Can you work these out from the model? Positions are in its coordinate system, mm. Face numbers are marked on the shaded views. A direction names the side the tool comes from. Round coordinates to 2 decimals unless told otherwise and drop trailing zeros. Write each loop counter-clockwise with the first axis right and the second up, starting at its lowest first coordinate (ties: lowest second). Pieces come first, ordered by that corner, then holes. Notation, with made-up numbers: M 75,-21 L 118,-21 A15 ccw 118,-6 Z; hole C 52.25,-2.75 d10. An arc over 180 degrees is marked long. Answer as a JSON object with one key per item and string values. Group by question number.
1) Suppose I cut it at A-A, the plane x = 0. Write out the boundary of the cut face in (y, z), and give its area (3 significant figures).
2) On a 3-axis mill with a long thin cutter (end or side, diameter ignored), from which of +Z, -Z, +X, -X, +Y, -Y can I reach the whole of each face in a straight line? I mean the marked faces 5, 6 and 7. Say none if no direction works.
3) Suppose I cut it at B-B, the plane y = -30.5. Write out the boundary of the cut face in (x, z), and give its area (3 significant figures).
4) If we mould it in two halves opening along X, with no side actions, what happens to the marked faces 1, 2, 3 and 4? For each: +X half, -X half, draft (parallel to the pull), parting line (faces both ways), or undercut.
5) Suppose I cut it at C-C, the plane x = 52.5. Write out the boundary of the cut face in (y, z), and give its area (3 significant figures).
6) Suppose I cut it at D-D, the plane z = 17.5. State how many separate pieces and enclosed holes the cut face has, and give its area (3 significant figures).
7) I'm going to push flat-ended pins straight in: pin 1 Ø2 at (y, z) = (-42, 16.5) entering from -X; pin 2 Ø5 at (x, z) = (66.5, 18) entering from +Y; pin 3 Ø4.5 at (y, z) = (-80.16, 12.5) entering from -X. Where does each tip first touch, or does it pass through?
8) Please list where these lines run through material, in increasing order: L1, parallel to X at y = -78, z = 15.5; L2, parallel to X at y = -1, z = 32; L3, parallel to Y at x = -38, z = 25.5. Write a range as [from, to].
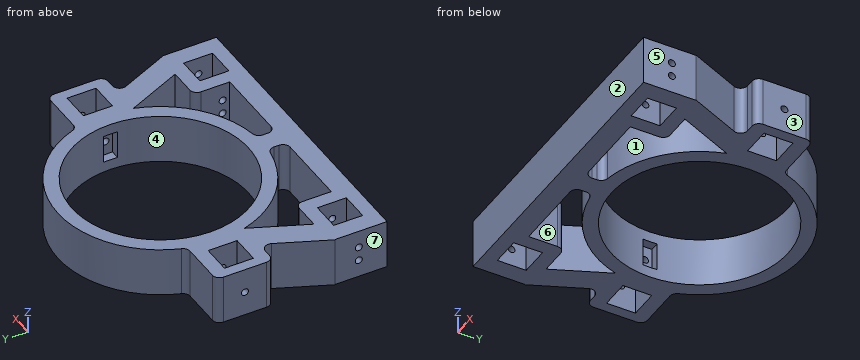
from build123d import *

# Parameters (mm, degrees)
SKETCH1_W                = 20.5
SKETCH1_H                = 20.5
SKETCH1_R                = 62.5
BOSS_EXTRUDE1_DEPTH      = 35
FILLET2_R                = 5
SKETCH2_W                = 20
SKETCH2_H                = 10
CUT_EXTRUDE2_DEPTH       = 7
SKETCH3_W                = 20
SKETCH3_H                = 10
CUT_EXTRUDE3_DEPTH       = 7
SKETCH4_W                = 35
SKETCH4_H                = 37
CUT_EXTRUDE4_DEPTH       = 10
SKETCH5_W                = 35
SKETCH5_H                = 37
CUT_EXTRUDE5_DEPTH       = 10
SKETCH6_W                = 35
SKETCH6_H                = 40.5
CUT_EXTRUDE8_DEPTH       = 2.5
SKETCH7_W                = 35
SKETCH7_H                = 40.5
CUT_EXTRUDE9_DEPTH       = 2.5
FILLET3_R                = 5
SKETCH8_R                = 2.5
CUT_EXTRUDE10_DEPTH      = 194
CUT_EXTRUDE10_DEPTH_BACK = 48
SKETCH9_R                = 2.5
CUT_EXTRUDE11_DEPTH      = 48
CUT_EXTRUDE11_DEPTH_BACK = 48
SKETCH10_R               = 2.5
CUT_EXTRUDE12_DEPTH      = 48
CUT_EXTRUDE12_DEPTH_BACK = 48


with BuildPart() as part:
    # Sketch1 → Boss-Extrude1 (new body)
    with BuildSketch(Plane.XY):
        with BuildLine():
            Line((117, -100.161277705), (117, -85.161277705))
            Line((117, -85.161277705), (88.226517383, -20.181680312))
            Line((88.226517383, -20.181680312), (108.734784021, -20.181680312))
            Line((108.734784021, -20.181680312), (108.734784021, 20.318319688))
            Line((108.734784021, 20.318319688), (69.594654141, 20.318319688))
            ThreePointArc((69.594654141, 20.318319688), (0, 72.5), (-69.594654141, 20.318319688))
            Line((-69.594654141, 20.318319688), (-108.734784021, 20.318319688))
            Line((-108.734784021, 20.318319688), (-108.734784021, -20.181680312))
            Line((-108.734784021, -20.181680312), (-88.226517383, -20.181680312))
            Line((-88.226517383, -20.181680312), (-117, -85.161277705))
            Line((-117, -85.161277705), (-117, -100.161277705))
            Line((-117, -100.161277705), (117, -100.161277705))
        make_face()
        with Locations((83.958397156, -79.911277705)):
            Rectangle(SKETCH1_W, SKETCH1_H, mode=Mode.SUBTRACT)
        with Locations((-83.958397156, -79.911277705)):
            Rectangle(SKETCH1_W, SKETCH1_H, mode=Mode.SUBTRACT)
        with BuildLine():
            Line((-63.708397156, -59.661277705), (-87.116280609, -59.661277705))
            Line((-87.116280609, -59.661277705), (-69.634400836, -20.181680312))
            ThreePointArc((-69.634400836, -20.181680312), (-46.29986484, -55.79043391), (-7, -72.161277705))
            Line((-7, -72.161277705), (-7, -85.161277705))
            Line((-7, -85.161277705), (-63.708397156, -85.161277705))
            Line((-63.708397156, -85.161277705), (-63.708397156, -59.661277705))
        make_face(mode=Mode.SUBTRACT)
        with BuildLine():
            Line((87.116280609, -59.661277705), (63.708397156, -59.661277705))
            Line((63.708397156, -59.661277705), (63.708397156, -85.161277705))
            Line((63.708397156, -85.161277705), (7, -85.161277705))
            Line((7, -85.161277705), (7, -72.161277705))
            ThreePointArc((7, -72.161277705), (46.29986484, -55.79043391), (69.634400836, -20.181680312))
            Line((69.634400836, -20.181680312), (87.116280609, -59.661277705))
        make_face(mode=Mode.SUBTRACT)
        with Locations((-88.484784021, 0.068319688)):
            Rectangle(SKETCH1_W, SKETCH1_H, mode=Mode.SUBTRACT)
        Circle(SKETCH1_R, mode=Mode.SUBTRACT)
        with Locations((88.484784021, 0.068319688)):
            Rectangle(SKETCH1_W, SKETCH1_H, mode=Mode.SUBTRACT)
    extrude(amount=BOSS_EXTRUDE1_DEPTH)

    # Fillet2
    fillet2_edges = [part.edges().sort_by_distance(p)[0] for p in [
        (-88.226517383, -20.181680312, 17.5),
        (-69.594654141, 20.318319688, 17.5),
        (69.594654141, 20.318319688, 17.5),
        (88.226517383, -20.181680312, 17.5),
        (7, -72.161277705, 17.5),
        (7, -85.161277705, 17.5),
        (63.708397156, -59.661277705, 17.5),
        (-63.708397156, -59.661277705, 17.5),
        (-7, -85.161277705, 17.5),
        (-7, -72.161277705, 17.5),
    ]]
    fillet(fillet2_edges, radius=FILLET2_R)

    # Sketch2 → Cut-Extrude2 (cut)
    with BuildSketch(Plane(origin=(61.7, 0, 0), x_dir=(0, 0, -1), z_dir=(1, 0, 0))):
        with Locations((-17.5, 0.068319688)):
            Rectangle(SKETCH2_W, SKETCH2_H)
    extrude(amount=CUT_EXTRUDE2_DEPTH, mode=Mode.SUBTRACT)

    # Sketch3 → Cut-Extrude3 (cut)
    with BuildSketch(Plane(origin=(-61.7, 0, 0), x_dir=(0, 0, -1), z_dir=(1, 0, 0))):
        with Locations((-17.5, 0.068319688)):
            Rectangle(SKETCH3_W, SKETCH3_H)
    extrude(amount=-CUT_EXTRUDE3_DEPTH, mode=Mode.SUBTRACT)

    # Sketch4 → Cut-Extrude4 (cut)
    with BuildSketch(Plane(origin=(117, 0, 0), x_dir=(0, 0, -1), z_dir=(1, 0, 0))):
        with Locations((-17.5, -81.661277705)):
            Rectangle(SKETCH4_W, SKETCH4_H)
    extrude(amount=-CUT_EXTRUDE4_DEPTH, mode=Mode.SUBTRACT)

    # Sketch5 → Cut-Extrude5 (cut)
    with BuildSketch(Plane.ZY.offset(117)):
        with Locations((17.5, -81.661277705)):
            Rectangle(SKETCH5_W, SKETCH5_H)
    extrude(amount=-CUT_EXTRUDE5_DEPTH, mode=Mode.SUBTRACT)

    # Sketch6 → Cut-Extrude8 (cut)
    with BuildSketch(Plane(origin=(108.734784021, 0, 0), x_dir=(0, 0, -1), z_dir=(1, 0, 0))):
        with Locations((-17.5, 0.068319688)):
            Rectangle(SKETCH6_W, SKETCH6_H)
    extrude(amount=-CUT_EXTRUDE8_DEPTH, mode=Mode.SUBTRACT)

    # Sketch7 → Cut-Extrude9 (cut)
    with BuildSketch(Plane.ZY.offset(108.734784021)):
        with Locations((17.5, 0.068319688)):
            Rectangle(SKETCH7_W, SKETCH7_H)
    extrude(amount=-CUT_EXTRUDE9_DEPTH, mode=Mode.SUBTRACT)

    # Fillet3
    fillet3_edges = [part.edges().sort_by_distance(p)[0] for p in [
        (106.234784021, 20.318319688, 17.5),
        (106.234784021, -20.181680312, 17.5),
        (-106.234784021, 20.318319688, 17.5),
        (-106.234784021, -20.181680312, 17.5),
    ]]
    fillet(fillet3_edges, radius=FILLET3_R)

    # Sketch8 → Cut-Extrude10 (cut, two sides)
    with BuildSketch(Plane(origin=(-68.7, 0, 0), x_dir=(0, 0, -1), z_dir=(1, 0, 0))) as cut_extrude10_sk:
        with Locations((-17.5, 0.068319688)):
            Circle(SKETCH8_R)
    extrude(amount=CUT_EXTRUDE10_DEPTH, mode=Mode.SUBTRACT)
    extrude(cut_extrude10_sk.sketch, amount=-CUT_EXTRUDE10_DEPTH_BACK, mode=Mode.SUBTRACT)

    # Sketch9 → Cut-Extrude11 (cut, two sides)
    with BuildSketch(Plane(origin=(-94.208397156, 0, 0), x_dir=(0, 0, -1), z_dir=(1, 0, 0))) as cut_extrude11_sk:
        with Locations((-22.5, -80.161277705)):
            Circle(SKETCH9_R)
        with Locations((-12.5, -80.161277705)):
            Circle(SKETCH9_R)
    extrude(amount=CUT_EXTRUDE11_DEPTH, mode=Mode.SUBTRACT)
    extrude(cut_extrude11_sk.sketch, amount=-CUT_EXTRUDE11_DEPTH_BACK, mode=Mode.SUBTRACT)

    # Sketch10 → Cut-Extrude12 (cut, two sides)
    with BuildSketch(Plane.ZY.offset(-94.208397156)) as cut_extrude12_sk:
        with Locations((12.5, -80.161277705)):
            Circle(SKETCH10_R)
        with Locations((22.5, -80.161277705)):
            Circle(SKETCH10_R)
    extrude(amount=CUT_EXTRUDE12_DEPTH, mode=Mode.SUBTRACT)
    extrude(cut_extrude12_sk.sketch, amount=-CUT_EXTRUDE12_DEPTH_BACK, mode=Mode.SUBTRACT)


solid = part.part
Results:
{
 "1": {"outline": "M -100.16,0 L -62.5,0 L -62.5,35 L -100.16,35 Z; M 62.5,0 L 72.5,0 L 72.5,35 L 62.5,35 Z", "area": "1,670 mm^2"},
 "2": {"face 5": "+Z, -Z, +X, -Y", "face 6": "+Z, -Z", "face 7": "+Z, -Z, -X, -Y"},
 "3": {"outline": "M -92.8,0 L -74.2,0 L -74.2,35 L -92.8,35 Z; M -65.77,0 L -54.55,0 L -54.55,35 L -65.77,35 Z; M 54.55,0 L 65.77,0 L 65.77,35 L 54.55,35 Z; M 74.2,0 L 92.8,0 L 92.8,35 L 74.2,35 Z", "area": "2,090 mm^2"},
 "4": {"face 1": "undercut", "face 2": "draft", "face 3": "+X half", "face 4": "undercut"},
 "5": {"outline": "M -100.16,0 L -85.16,0 L -85.16,35 L -100.16,35 Z; M -50,0 L -33.91,0 L -33.91,35 L -50,35 Z; M 33.91,0 L 50,0 L 50,35 L 33.91,35 Z", "area": "1,650 mm^2"},
 "6": {"separate pieces": "2", "enclosed holes": "4", "area": "12,200 mm^2"},
 "7": {"pin 1": "x = -98.33", "pin 2": "y = 34.06", "pin 3": "x = -7.53"},
 "8": {"L1": "[-107, -94.21], [-73.71, -63.71], [-7, 7], [63.71, 73.71], [94.21, 107]", "L2": "[-106.23, -98.73], [-78.23, -62.49], [62.49, 78.23], [98.73, 106.23]", "L3": "[-100.16, -85.16], [-61.74, -49.62], [49.62, 61.74]"}
}
